```python
from build123d import *

# Parameters (mm, degrees)
SKETCH1_R           = 20
BOSS_EXTRUDE1_DEPTH = 5
SKETCH2_R           = 7.5
BOSS_EXTRUDE2_DEPTH = 13
CUT_EXTRUDE1_DEPTH  = 18
SKETCH4_R           = 2
CUT_EXTRUDE2_DEPTH  = 18


with BuildPart() as part:
    # Sketch1 → Boss-Extrude1 (new body)
    with BuildSketch(Plane.XY):
        Circle(SKETCH1_R)
    extrude(amount=BOSS_EXTRUDE1_DEPTH)

    # Sketch2 → Boss-Extrude2 (add)
    with BuildSketch(Plane.XY.offset(5)):
        Circle(SKETCH2_R)
    extrude(amount=BOSS_EXTRUDE2_DEPTH)

    # Sketch3 → Cut-Extrude1 (cut)
    with BuildSketch(Plane.XY.offset(18)):
        with BuildLine():
            Line((-2.645751311, 3), (2.645751311, 3))
            ThreePointArc((2.645751311, 3), (0, -4), (-2.645751311, 3))
        make_face()
    extrude(amount=-CUT_EXTRUDE1_DEPTH, mode=Mode.SUBTRACT)

    # Sketch4 → Cut-Extrude2 (cut)
    with BuildSketch(Plane.XY.offset(5)):
        with Locations((0, 15)):
            Circle(SKETCH4_R)
        with Locations((15, 0)):
            Circle(SKETCH4_R)
        with Locations((0, -15)):
            Circle(SKETCH4_R)
        with Locations((-15, 0)):
            Circle(SKETCH4_R)
    extrude(amount=-CUT_EXTRUDE2_DEPTH, mode=Mode.SUBTRACT)


solid = part.part
```
Can you work these out from the model? Positions are in its coordinate system, mm. A direction names the side the tool comes from. Coordinates: 2 decimals unless noted, no trailing zeros. Loops run counter-clockwise (first coordinate to the right, second up) from the corner with the lowest first, then second, coordinate; pieces in that order, holes last.
Item 1: If we mould it in two halves opening along Y, with no side actions, what happens to faces 4 (the face through (-0.3, -4.2, 0)), 5 (the face through (13.4, -1.2, 2.5)), 6 (the face through (0, -4, 9)), 7 (the face through (-4.336, -19.524, 2.465))? For each: released by +Y, released by -Y, zero draft, split by the parting line, or undercut.
Answers below:
face 4: zero draft
face 5: undercut
face 6: undercut
face 7: split by the parting line
Item 2: Suppose I cut it at B-B (y = -13.5). Please give me the cut outline in (x, z), then the cut area to 3 significant figures.
Answers below:
outline: (-14.76, 0) - (-1.32, 0) - (-1.32, 5) - (-14.76, 5) - close; (1.32, 0) - (14.76, 0) - (14.76, 5) - (1.32, 5) - close
area: 134 mm2
Item 3: Suppose I cut it at C-C (z = 1.75). Please give me the cut outline in (x, y).
Answers below:
outline: circle Ø40 at (0, 0); hole circle Ø4 at (-15, 0); hole (-2.65, 3) arc R4 ccw (long way) to (2.65, 3) - close; hole circle Ø4 at (0, -15); hole circle Ø4 at (0, 15); hole circle Ø4 at (15, 0)
Item 4: Which directions (+Z, -Z, +X, -X, +Y, -Y) give clear straight access to the entire face, cutting with the end or side of a thin tool? Please do faces 1 (the face through (-0.1, 3.4, 18)), 2 (the face through (0, -9, 5)), 3 (the face through (0, 3, 9)).
Answers below:
face 1: +Z, +X, -X, +Y, -Y
face 2: +Z
face 3: +Z, -Z
Item 5: Suppose I cut it at D-D (x = -15). Please give me the cut outline in (y, z).
Answers below:
outline: (-13.23, 0) - (-2, 0) - (-2, 5) - (-13.23, 5) - close; (2, 0) - (13.23, 0) - (13.23, 5) - (2, 5) - close
Item 6: Please list where these lines run through material, in increasing order: L1, parallel to Z at x = -13.5, y = -8; L2, parallel to X at y = -0.5, z = 3.75; L3, parallel to X at y = 2, z = 5.75.
Answers below:
L1: z = 0 to 5
L2: x = -19.99 to -16.94, -13.06 to -3.97, 3.97 to 13.06, 16.94 to 19.99
L3: x = -7.23 to -3.46, 3.46 to 7.23
Item 7: Suppose I cut it at A-A (x = 0). Please give me the cut outline in (y, z), then the cut area to 3 significant figures.
Answers below:
outline: (-20, 0) - (-17, 0) - (-17, 5) - (-20, 5) - close; (-13, 0) - (-4, 0) - (-4, 18) - (-7.5, 18) - (-7.5, 5) - (-13, 5) - close; (3, 0) - (13, 0) - (13, 5) - (7.5, 5) - (7.5, 18) - (3, 18) - close; (17, 0) - (20, 0) - (20, 5) - (17, 5) - close
area: 229 mm2
Item 8: I'm going to push flat-ended pins straight in: pin 1 (4.5 mm diameter, centred on x = -15, y = 0, fed in from +Z); pin 2 (2 mm diameter, centred on y = -4.5, z = 9.5, fed in from -X); pin 3 (1 mm diameter, centred on y = 15, z = 3.5, fed in from -X) (3 decimals); pin 4 (6.5 mm diameter, centred on x = 0, y = 15, fed in from -Z). Where does each tip first touch, or does it pass through?
Answers below:
pin 1: stops at z = 5
pin 2: stops at x = -6.63
pin 3: stops at x = -13.775
pin 4: stops at z = 0
